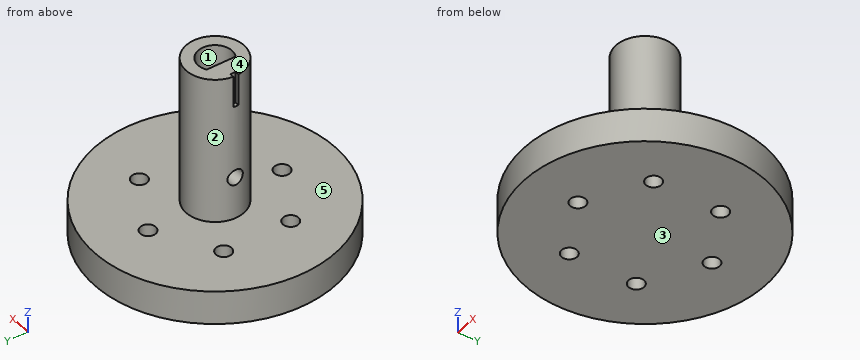
Autodesk Inventor part; units mm, degrees
ref_plane "Plano de trabajo2" through (-6.8425, 0, 8) normal (1, 0, 0) x (0, 1, 0)
ref_plane "Plano de trabajo3" through (0, 22.5, 15) normal (0, 0, -1) x (-1, 0, 0)
ref_plane "Plano de trabajo4" through (0, 11, 8) normal (0, 0, -1) x (-1, 0, 0)
sketch "Boceto1" plane through (0, 0, 0) normal (0, 0, 1) x (1, 0, 0)
  circle A0 centre (0, 0) radius 28.5
  dimension "DiametroJunta" = 57
extrude "Extrusión1" add sketch "Boceto1" along normal blind 8
sketch "Boceto2" plane through (0, 0, 8) normal (0, 0, 1) x (1, 0, 0)
  circle A0 centre (0, 0) radius 6.8425
  dimension "DiametroEje" = 13.685
extrude "Extrusión2" add sketch "Boceto2" along normal blind 35
sketch "Boceto3" plane through (0, 0, 43) normal (0, 0, 1) x (1, 0, 0)
  arc A0 (-2, -3.4641) -> (-2, 3.4641) centre (0, 0) ccw
  line L0 (-2, 3.4641) -> (-2, -3.4641)
  circle A1 centre (0, 0) radius 6.8425
  point P0 (2, -3.4641)
  point P1 (2, 3.4641)
  dimension "DiametroEntrada" = 8
  dimension "d21" = 2
extrude "Extrusión3" cut sketch "Boceto3" against normal blind 34.5 contours L0 A0
ref_plane "Plano de trabajo1" through (6.8425, 0, 8) normal (1, 0, 0) x (0, 1, 0)
ref_plane "Plano de trabajo2" through (-6.8425, 0, 8) normal (1, 0, 0) x (0, 1, 0)
sketch "Boceto5" plane through (-6.8425, 0, 8) normal (1, 0, 0) x (0, 1, 0)
  line L0 (6.8425, 35) -> (-6.8425, 35)
  line L1 (0, 35) -> (0, 10)
  circle A0 centre (0, 10) radius 1.4978
  line L2 (-0.6, 27.4718) -> (0.6, 27.4718)
  line L3 (0.6, 27.4718) -> (0.6, 35)
  line L4 (0.6, 35) -> (-0.6, 35)
  line L5 (-0.6, 35) -> (-0.6, 27.4718)
  line L6 (-0.6, 27.4718) -> (0.6, 35) construction
  line L7 (0.6, 27.4718) -> (-0.6, 35) construction
  point P0 (0, -8)
  point P1 (0, 31.2359)
  dimension "d54" = 25
  dimension "d91" = 1.2
hole "Agujero2" at (-6.8425, 0, 18) direction (1, 0, 0) diameter 3.6881 depth 6 tip angle 118
sketch "Boceto7" plane through (0, 0, 0) normal (0, 0, -1) x (-1, 0, 0)
  arc A0 (2, 3.4641) -> (2, -3.4641) centre (0, 0) ccw
  circle A1 centre (0, 16) radius 5
  dimension "d35" = 10
  dimension "d49" = 16
ref_plane "Plano de trabajo3" through (0, 22.5, 15) normal (0, 0, -1) x (-1, 0, 0)
ref_plane "Plano de trabajo4" through (0, 11, 8) normal (0, 0, -1) x (-1, 0, 0)
sketch "Boceto9" plane through (0, 11, 8) normal (0, 0, -1) x (-1, 0, 0)
  circle A0 centre (0, 0) radius 2.5
  point P0 (0, -11)
  dimension "d70" = 5
hole "Agujero6" at (0, 16, 0) direction (0, 0, 1) diameter 3.6881 depth 13
pattern_circular "Patrón circular6" count 6 over 360 about axis through (0, 0, 8) along (0, 0, 1) of "Agujero6"
extrude "Extrusión6" add sketch "Boceto5" along normal blind 1 contours L3 L2 L1 L0 | L1 L2 L5 L0
extrude "Extrusión7" cut sketch "Boceto5" along normal blind 1 contours L3 L2 L1 L0 | L1 L2 L5 L0
properties part number "E_01" material "PETG"
CAD build for the part. Positions are in the model's coordinates, mm. Face numbers are marked on the shaded views. A direction names the side the tool comes from. Coordinates: 2 decimals unless noted, no trailing zeros. Order: outer loops, then holes, each group sorted by start corner. A loop starts at its lowest first (then second) coordinate and runs counter-clockwise, first axis right, second up. Notation, with made-up numbers: (12.25, -6) -> (50.25, -6) arc R10 ccw to (50.25, 8) -> close; hole circle Ø11 at (6, 58.25). An arc over 180 degrees is marked (long way). Use one line per item in the form item = value. Start each with the question number.
1) Band-saw the part on B-B on y = -16. Give the cut face in (x, z).
2) Band-saw the part on D-D on z = 22.5. Give the cut face in (x, y) (1 decimal).
3) Drop flat-ended pins along their axis: pin 1 (12 mm diameter, centred on x = 5.5, y = -15, fed in from +Z); pin 2 (5 mm diameter, centred on x = -13.86, y = 8, fed in from -Z); pin 3 (3.5 mm diameter, centred on y = 0.5, z = 28, fed in from +X); pin 4 (3 mm diameter, centred on y = 6, z = 11, fed in from -X). Give the stop position or say it passes through.
4) Band-saw the part on C-C on y = -8. Give the cut face in (x, z).
5) Band-saw the part on A-A on x = 0. Give the cut face in (y, z).
6) Drill centre lines: L1, parallel to Y at x = 0.5, z = 3; L2, parallel to X at y = 8, z = 4.75; L3, parallel to Z at x = -1, y = 23. Where is each one in solid material? Low to high. Write a range as [from, to].
7) Tool access for the marked faces 4 and 5: list every direction of +Z, -Z, +X, -X, +Y, -Y with a clear straight run to the whole face (end or side of a thin tool).
8) Pull direction Y, two halves, no side cores. Call the marked faces 1, 2 and 3: +Y half, -Y half, draft (parallel to the pull), parting line (faces both ways), or undercut.
Entries:
q1.outline = (-23.58, 0) -> (-1.84, 0) -> (-1.84, 8) -> (-23.58, 8) -> close; (1.84, 0) -> (23.58, 0) -> (23.58, 8) -> (1.84, 8) -> close
q2.outline = circle Ø13.7 at (0, 0); hole (-2, -3.5) arc R4 ccw (long way) to (-2, 3.5) -> close
q3.pin_1 = 8
q3.pin_2 = 0
q3.pin_3 = 6.84
q3.pin_4 = -5.15
q4.outline = (-27.35, 0) -> (-15.7, 0) -> (-15.7, 8) -> (-27.35, 8) -> close; (-12.01, 0) -> (12.01, 0) -> (12.01, 8) -> (-12.01, 8) -> close; (15.7, 0) -> (27.35, 0) -> (27.35, 8) -> (15.7, 8) -> close
q5.outline = (-28.5, 0) -> (-17.84, 0) -> (-17.84, 8) -> (-28.5, 8) -> close; (-14.16, 0) -> (14.16, 0) -> (14.16, 8) -> (6.84, 8) -> (6.84, 43) -> (4, 43) -> (4, 8.5) -> (-4, 8.5) -> (-4, 43) -> (-6.84, 43) -> (-6.84, 8) -> (-14.16, 8) -> close; (17.84, 0) -> (28.5, 0) -> (28.5, 8) -> (17.84, 8) -> close
q6.L1 = [-28.5, -17.77], [-14.23, 14.23], [17.77, 28.5]
q6.L2 = [-27.35, -15.7], [-12.01, 12.01], [15.7, 27.35]
q6.L3 = [0, 8]
q7.face_4 = +Z, +X, -X, +Y, -Y
q7.face_5 = +Z
q8.face_1 = undercut
q8.face_2 = parting line
q8.face_3 = draft
